Input: dimensioned drawing with shaded views. Units: mm. Origin: part minimum x, y, z. A direction names the side the tool comes from. Give positions to 0.01 mm unless a question says otherwise; leave off trailing zeros. Order: outer loops, then holes, each group sorted by start corner. A loop starts at its lowest first (then second) coordinate and runs counter-clockwise, first axis right, second up. Notation, with made-up numbers: (21.25, 25.5) - (27.25, 25.5) arc R21 ccw to (27.25, 50.5) - close; hole circle Ø8 at (-23, 18). An arc over 180 degrees is marked (long way). Answer as CSV lines item,"result".
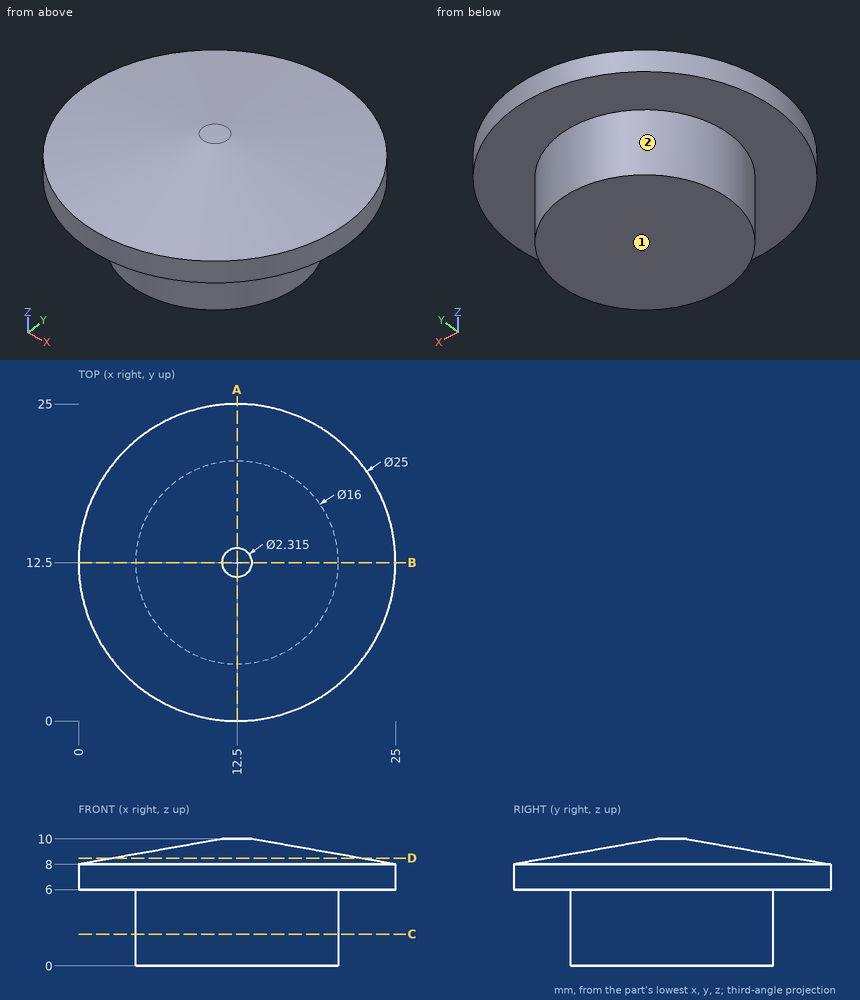
(1) Access query for the marked faces 1 and 2. Directions: +Z, -Z, +X, -X, +Y, -Y. A direction counts if a zero-diameter tool reaches every point of the face in a straight line with its end or side. Return the directions, or none.
Completed:
face 1,"-Z, +X, -X, +Y, -Y"
face 2,"-Z"
(2) Ray query, line 1 (Z direction, x = 11, y = 2); line 2 (X direction, y = 9.75, z = 1.5); line 3 (X direction, y = 10.5, z = 2.5). Return the intervals inside material, ascending. Write a range as from..to.
Completed:
line 1,"6..8.33"
line 2,"4.99..20.01"
line 3,"4.75..20.25"
(3) Contact query for flat-ended pins moving along their axis: pin 1 (6 mm diameter, centred on y = 9.5, z = 4.5, fed in from -X); pin 2 (1.5 mm diameter, centred on x = 22.5, z = 6.5, fed in from -Y); pin 3 (4 mm diameter, centred on x = 22, z = 7, fed in from -Y). Output: stop coordinate, or through.
Completed:
pin 1,"x = 0.01"
pin 2,"y = 4.09"
pin 3,"y = 2.5"
(4) Cut plane A-A (x = 12.5). Return loops of the section in (y, z).
Completed:
outline,"(0, 6) - (4.5, 6) - (4.5, 0) - (20.5, 0) - (20.5, 6) - (25, 6) - (25, 8) - (13.66, 10) - (11.34, 10) - (0, 8) - close"
(5) Cut plane D-D (z = 8.5). Return loops of the section in (x, y), then the cut area to 3 significant figures.
Completed:
outline,"circle Ø19.33 at (12.5, 12.5)"
area,"293 mm²"
(6) Cut plane C-C (z = 2.5). Return loops of the section in (x, y), then the cut area to 3 significant figures.
Completed:
outline,"circle Ø16 at (12.5, 12.5)"
area,"201 mm²"
